CAD build for the part. Positions are in the model's coordinates, mm. A direction names the side the tool comes from. Coordinates: 2 decimals unless noted, no trailing zeros. Loops run counter-clockwise (first coordinate to the right, second up) from the corner with the lowest first, then second, coordinate; pieces in that order, holes last. Notation, with made-up numbers: (61.25, 18.5) -> (90.25, 18.5) arc R20 ccw to (90.25, 26.5) -> close; hole circle Ø8 at (12.25, 42.5). An arc over 180 degrees is marked (long way). Write each question's results on one line, items separated by ' | '.
```python
from build123d import *

# Parameters (mm, degrees)
F0_R     = 4
F1_DEPTH = 40
F2_W     = 12.5
F2_H     = 30
F3_DEPTH = 70
F4_R     = 2.5
F5_DEPTH = 25


with BuildPart() as f1:
    # F0 (on Top) → F1 (new body)
    with BuildSketch(Plane.XY):
        with BuildLine():
            Line((-35, 22), (-35, -22))
            Line((-35, -22), (35, -22))
            Line((35, -22), (35, 22))
            ThreePointArc((35, 22), (0, 10.4279927909), (-35, 22))
        make_face()
        with Locations((-27, -15)):
            Circle(F0_R, mode=Mode.SUBTRACT)
        with Locations((0, -15)):
            Circle(F0_R, mode=Mode.SUBTRACT)
        with Locations((27, -15)):
            Circle(F0_R, mode=Mode.SUBTRACT)
    extrude(amount=F1_DEPTH)

    # F2 (on face) → F3 (cut)
    with BuildSketch(Plane.YZ.offset(35)):
        with Locations((-15.75, 15)):
            Rectangle(F2_W, F2_H)
    extrude(amount=-F3_DEPTH, mode=Mode.SUBTRACT)

    # F4
    f4_edges = [f1.edges().sort_by_distance(p)[0] for p in [
        (35, 22, 20),
        (-35, 22, 20),
    ]]
    fillet(f4_edges, radius=F4_R)

    # F5 (cut): a face of the model
    f5_faces = [f1.faces().sort_by_distance(p)[0] for p in [
        (0, 2.4481548638, 0),
    ]]
    extrude(f5_faces, amount=-F5_DEPTH, mode=Mode.SUBTRACT)


solid = f1.part
```
Q1. Wall check: L1, parallel to X at y = -15, z = 33.75; L2, parallel to Y at x = 0, z = 33.5; L3, parallel to Z at x = -20, y = -17.5. Give the ranges that are in metal, low to high. Write a range as from..to.
Results are:
L1: -35..-31, -23..-4, 4..23, 31..35 | L2: -22..-19, -11..10.43 | L3: 30..40
Q2. Cut at D-D on x = -15. Write the cut outline in (y, z), and give its area (3 significant figures).
Results are:
outline: (-22, 30) -> (-9.5, 30) -> (-9.5, 25) -> (12.38, 25) -> (12.38, 40) -> (-22, 40) -> close | area: 453 mm^2
Q3. Cut at C-C on x = -27. Write the cut outline in (y, z), and give its area (3 significant figures).
Results are:
outline: (-22, 30) -> (-19, 30) -> (-19, 40) -> (-22, 40) -> close; (-11, 30) -> (-9.5, 30) -> (-9.5, 25) -> (17, 25) -> (17, 40) -> (-11, 40) -> close | area: 443 mm^2
Q4. Cut at A-A on y = -15. Write the cut outline in (x, z), and give its area (3 significant figures).
Results are:
outline: (-35, 30) -> (-31, 30) -> (-31, 40) -> (-35, 40) -> close; (-23, 30) -> (-4, 30) -> (-4, 40) -> (-23, 40) -> close; (4, 30) -> (23, 30) -> (23, 40) -> (4, 40) -> close; (31, 30) -> (35, 30) -> (35, 40) -> (31, 40) -> close | area: 460 mm^2
Q5. Which spindle directions (+Z, -Z, +X, -X, +Y, -Y) get a long thin tool onto all of the face, cutting with end or side? Do faces 1 (the flat face through (0, -20, 30)), 2 (the flat face through (0, -5, 40)). Say none if no direction does.
Results are:
face 1: -Z, +X, -X, -Y | face 2: +Z, +X, -X, +Y, -Y
Q6. Pull direction X, two halves, no side cores. Call faces 3 (the cylindrical face through (-29.95, -12.3, 34.93)), 4 (the cylindrical face through (24.05, -12.3, 34.93)), 5 (the flat face through (0, -9.5, 27)), 6 (the flat face through (35, -3, 32)): +X half, -X half, draft (parallel to the pull), parting line (faces both ways), or undercut.
Results are:
face 3: undercut | face 4: undercut | face 5: draft | face 6: +X half
Q7. Cut at B-B on z = 36.5. Write the cut outline in (x, y), and give its area (3 significant figures).
Results are:
outline: (-35, -22) -> (35, -22) -> (35, 17.27) arc R2.5 ccw to (31.17, 19.39) arc R58.72 cw to (-31.17, 19.39) arc R2.5 ccw to (-35, 17.27) -> close; hole circle Ø8 at (-27, -15); hole circle Ø8 at (0, -15); hole circle Ø8 at (27, -15) | area: 2,370 mm^2
Q8. Drop flat-ended pins along their axis: pin 1 (9 mm diameter, centred on x = 0, y = -15, fed in from +Z); pin 2 (1.5 mm diameter, centred on x = 14, z = 27.5, fed in from -Y); pin 3 (4 mm diameter, centred on x = -4, y = -12, fed in from -Z). Give the stop position or say it passes through.
Results are:
pin 1: z = 40 | pin 2: y = -9.5 | pin 3: z = 30
